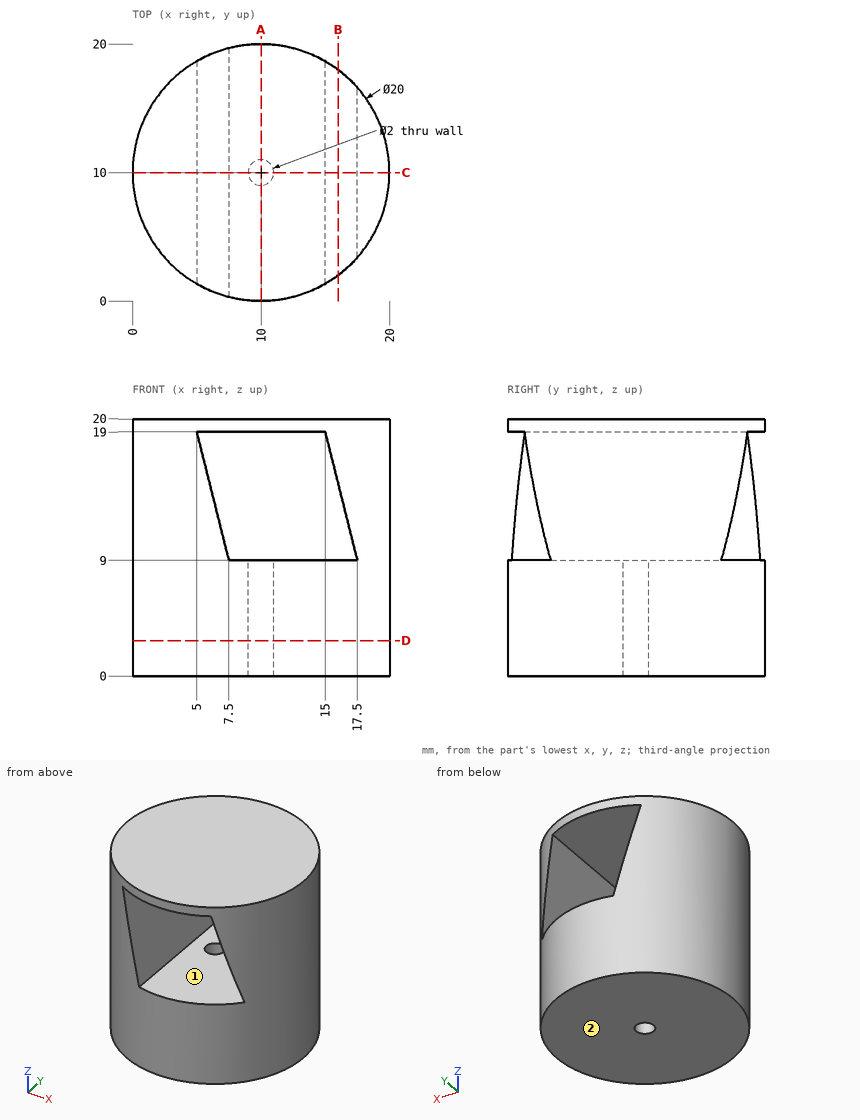
Here's the drawing with two shaded views (mm, measured from the low corner). I have some questions. A direction names the side the tool comes from. Give positions to 0.01 mm unless a question says otherwise; leave off trailing zeros. Loops run counter-clockwise (first coordinate to the right, second up) from the corner with the lowest first, then second, coordinate; pieces in that order, holes last. Notation, with made-up numbers: M 73.5,31 L 108.5,31 A15 cw 108.5,58 Z; hole C -11.5,86 d4. An arc over 180 degrees is marked long. Use one line per item in the form item = value. Start each with the question number.
(1) On a 3-axis mill with a long thin cutter (end or side, diameter ignored), from which of +Z, -Z, +X, -X, +Y, -Y can I reach the whole of each face in a straight line? I mean the marked faces 1 and 2. Say none if no direction works.
(2) I want a section at C-C, the plane y = 10. Write out the boundary of the cut face in (x, z).
(3) I want a section at D-D, the plane z = 2.75. Write out the boundary of the cut face in (x, y), and give its area (3 significant figures).
(4) I want a section at A-A, the plane x = 10. Write out the boundary of the cut face in (y, z), and give its area (3 significant figures).
(5) Please list where these lines run through material, in increasing order: line 1 (Z direction, x = 10.25, y = 1.5); line 2 (Y direction, x = 10, z = 5.75); line 3 (X direction, y = 15, z = 13).
(6) I want a section at B-B, the plane x = 16. Write out the boundary of the cut face in (y, z).
(7) I'm going to push flat-ended pins straight in: P1, Ø12, axis at y = 18, z = 17.5, coming from the -X side; P2, Ø12, axis at y = 17, z = 15, coming from the -X side; P3, Ø2, axis at x = 3.5, z = 3.5, coming from the +Y side. Where does each tip first touch, or does it pass through?
Worked out:
q1.face_1 = +Y, -Y
q1.face_2 = -Z, +X, -X, +Y, -Y
q2.outline = M 0,0 L 9,0 L 9,9 L 7.5,9 L 5,19 L 15,19 L 17.5,9 L 11,9 L 11,0 L 20,0 L 20,20 L 0,20 Z
q3.outline = C 10,10 d20; hole C 10,10 d2
q3.area = 311 mm²
q4.outline = M 0,0 L 9,0 L 9,9 L 0,9 Z; M 0,19 L 20,19 L 20,20 L 0,20 Z; M 11,0 L 20,0 L 20,9 L 11,9 Z
q4.area = 182 mm²
q5.line_1 = 0 to 9, 19 to 20
q5.line_2 = 0 to 9, 11 to 20
q5.line_3 = 1.34 to 6.5, 16.5 to 18.66
q6.outline = M 2,0 L 18,0 L 18,9 L 2,9 Z; M 2,15 L 18,15 L 18,20 L 2,20 Z
q7.P1 = 0.2
q7.P2 = 0.05
q7.P3 = 18.35
